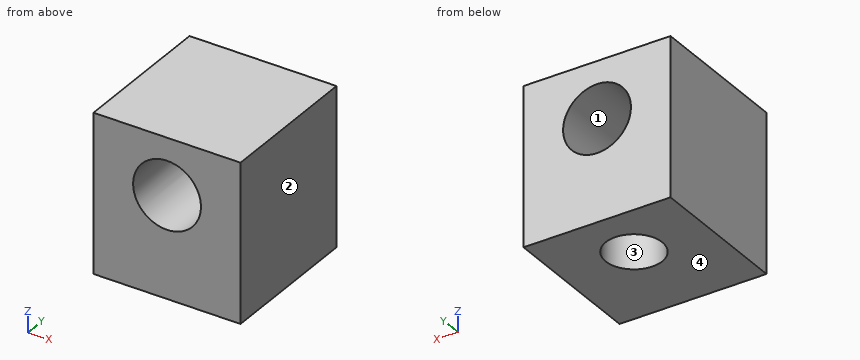
```python
from build123d import *

# Parameters (mm, degrees)
SKETCH1_W                 = 13
SKETCH1_H                 = 13
BOSS_EXTRUDE1_DEPTH       = 14
F_6_0MM_DOWEL_HOLE1_D     = 6
F_6_0MM_DOWEL_HOLE1_DEPTH = 13
M6X1_0_TAPPED_HOLE6_D     = 5
M6X1_0_TAPPED_HOLE6_DEPTH = 7
M6X1_0_TAPPED_HOLE6_TIP   = 1.502151548


with BuildPart() as part:
    # Sketch1 → Boss-Extrude1 (new body)
    with BuildSketch(Plane.XY):
        Rectangle(SKETCH1_W, SKETCH1_H)
    extrude(amount=BOSS_EXTRUDE1_DEPTH)

    # Ø6.0mm Dowel Hole1
    with Locations(Plane(origin=(0, 6.5, 0), x_dir=(1, 0, 0), z_dir=(0, 1, 0))):
        with Locations((0, -9)):
            Hole(F_6_0MM_DOWEL_HOLE1_D / 2, depth=F_6_0MM_DOWEL_HOLE1_DEPTH)

    # M6x1.0 Tapped Hole6
    with Locations(Plane(origin=(0, 0, 0), x_dir=(-1, 0, 0), z_dir=(0, 0, -1))):
        with Locations((0, 1.5)):
            Hole(M6X1_0_TAPPED_HOLE6_D / 2, depth=M6X1_0_TAPPED_HOLE6_DEPTH)
            with Locations((0, 0, -(M6X1_0_TAPPED_HOLE6_DEPTH + M6X1_0_TAPPED_HOLE6_TIP / 2))):  # 118° drill point
                Cone(0, M6X1_0_TAPPED_HOLE6_D / 2, M6X1_0_TAPPED_HOLE6_TIP, mode=Mode.SUBTRACT)


solid = part.part
```
Build history of the part. All positions in model axes, mm. Face numbers are marked on the shaded views. Give positions to 0.01 mm unless a question says otherwise; leave off trailing zeros. Loops run counter-clockwise (first coordinate to the right, second up) from the corner with the lowest first, then second, coordinate; pieces in that order, holes last.
1) Band-saw the part on D-D on y = 5.5. List the corners of the cut face in (x, z), then the cut area to 3 significant figures.
Values follow:
outline: (-6.5, 0) - (6.5, 0) - (6.5, 14) - (-6.5, 14) - close; hole circle Ø6 at (0, 9)
area: 154 mm2
2) Band-saw the part on A-A on x = -1. List the corners of the cut face in (y, z).
Values follow:
outline: (-6.5, 0) - (-0.79, 0) - (-0.79, 6.17) - (-6.5, 6.17) - close; (-6.5, 11.83) - (6.5, 11.83) - (6.5, 14) - (-6.5, 14) - close; (3.79, 0) - (6.5, 0) - (6.5, 6.17) - (3.79, 6.17) - close
3) Two-plate mould, pull along X, no slides. Class the marked faces 1, 2, 3 and 4: released by +X, released by -X, zero draft, split by the parting line, or undercut.
Values follow:
face 1: undercut
face 2: released by +X
face 3: undercut
face 4: zero draft
4) Drop a flat-ended pin along its axis: P1, Ø4, axis at x = 0, y = 1.5, coming from the -Z side. Give the stop position or say it passes through.
Values follow:
P1: stops at z = 11.24
5) Band-saw the part on C-C on z = 4.75. List the corners of the cut face in (x, y), then the cut area to 3 significant figures.
Values follow:
outline: (-6.5, -6.5) - (6.5, -6.5) - (6.5, 6.5) - (-6.5, 6.5) - close; hole circle Ø5 at (0, 1.5)
area: 149 mm2
6) Probe line 1 along Z through (x, y) = (0, -2.75); line 2 along X through (y, z) = (-0.5, 9); line 3 along Y through (x, z) = (0, 3.5). List the from-to ranges inside material, lowest first.
Values follow:
line 1: z = 0 to 6, 12 to 14
line 2: x = -6.5 to -3, 3 to 6.5
line 3: y = -6.5 to -1, 4 to 6.5
7) Band-saw the part on B-B on z = 9. List the corners of the cut face in (x, y), then the cut area to 3 significant figures.
Values follow:
outline: (-6.5, -6.5) - (-3, -6.5) - (-3, 6.5) - (-6.5, 6.5) - close; (3, -6.5) - (6.5, -6.5) - (6.5, 6.5) - (3, 6.5) - close
area: 91.0 mm2
